Could you check a few things on this model? Use its own coordinates, in mm. Give positions to 0.01 mm unless a question says otherwise; leave off trailing zeros. Write each loop counter-clockwise with the first axis right and the second up, starting at its lowest first coordinate (ties: lowest second). Pieces come first, ordered by that corner, then holes. Notation, with made-up numbers: M 35,-31.75 L 64,-31.75 A7 ccw 64,-23.75 Z; hole C 28,-17 d5. An arc over 180 degrees is marked long. Answer as CSV lines item,"result". Start each with the question number.
from build123d import *

# Parameters (mm, degrees)
SKETCH1_R          = 3.4
BASE_EXTRUDE_DEPTH = 6


with BuildPart() as part:
    # Sketch1 → Base-Extrude (new body)
    with BuildSketch(Plane.XY):
        with BuildLine():
            Line((-20, 0), (20, 0))
            ThreePointArc((20, 0), (23.535533906, 1.464466094), (25, 5))
            Line((25, 5), (25, 130.441190629))
            ThreePointArc((25, 130.441190629), (24.095760221, 133.309072811), (21.710100717, 135.139653733))
            Line((21.710100717, 135.139653733), (-18.289899283, 149.698463104))
            ThreePointArc((-18.289899283, 149.698463104), (-22.867882182, 149.095760221), (-25, 145))
            Line((-25, 145), (-25, 5))
            ThreePointArc((-25, 5), (-23.535533906, 1.464466094), (-20, 0))
        make_face()
        with Locations((0, 120)):
            Circle(SKETCH1_R, mode=Mode.SUBTRACT)
        with Locations((0, 20)):
            Circle(SKETCH1_R, mode=Mode.SUBTRACT)
    extrude(amount=BASE_EXTRUDE_DEPTH)


solid = part.part
1. Imagine slicing it at D-D, the plane y = 18.5. Please give me the cut outline in (x, z).
2. Thinking about a two-plate mould opening in X: for faces 1 (the cylindrical face through (-0.44, 123.37, 2.96)), 2 (the cylindrical face through (24.1, 133.3, 3)), 3 (the cylindrical face through (-23, 149, 3)), which applies, pulls with the +X half, pulls with the -X half, needs draft (parallel to the pull), parting line crosses it, or undercut?
3. Imagine slicing it at C-C, the plane x = 0. Please give me the cut outline in (y, z).
4. Imagine slicing it at B-B, the plane z = 5. Please give me the cut outline in (x, y).
5. Please list where these lines run through material, in increasing order: line 1 (Y direction, x = 0, z = 1.9); line 2 (Y direction, x = -2.5, z = 3.05); line 3 (X direction, y = 21, z = 4.9).
6. Imagine slicing it at A-A, the plane y = 120. Please give me the cut outline in (x, z), plus the area to 3 significant figures.
Solutions:
1,outline,"M -25,0 L -3.05,0 L -3.05,6 L -25,6 Z; M 3.05,0 L 25,0 L 25,6 L 3.05,6 Z"
2,face 1,"undercut"
2,face 2,"pulls with the +X half"
2,face 3,"parting line crosses it"
3,outline,"M 0,0 L 16.6,0 L 16.6,6 L 0,6 Z; M 23.4,0 L 116.6,0 L 116.6,6 L 23.4,6 Z; M 123.4,0 L 143.04,0 L 143.04,6 L 123.4,6 Z"
4,outline,"M -25,5 A5 ccw -20,0 L 20,0 A5 ccw 25,5 L 25,130.44 A5 ccw 21.71,135.14 L -18.29,149.7 A5 ccw -25,145 Z; hole C 0,20 d6.8; hole C 0,120 d6.8"
5,line 1,"0 to 16.6, 23.4 to 116.6, 123.4 to 143.04"
5,line 2,"0 to 17.7, 22.3 to 117.7, 122.3 to 143.95"
5,line 3,"-25 to -3.25, 3.25 to 25"
6,outline,"M -25,0 L -3.4,0 L -3.4,6 L -25,6 Z; M 3.4,0 L 25,0 L 25,6 L 3.4,6 Z"
6,area,"259 mm²"
